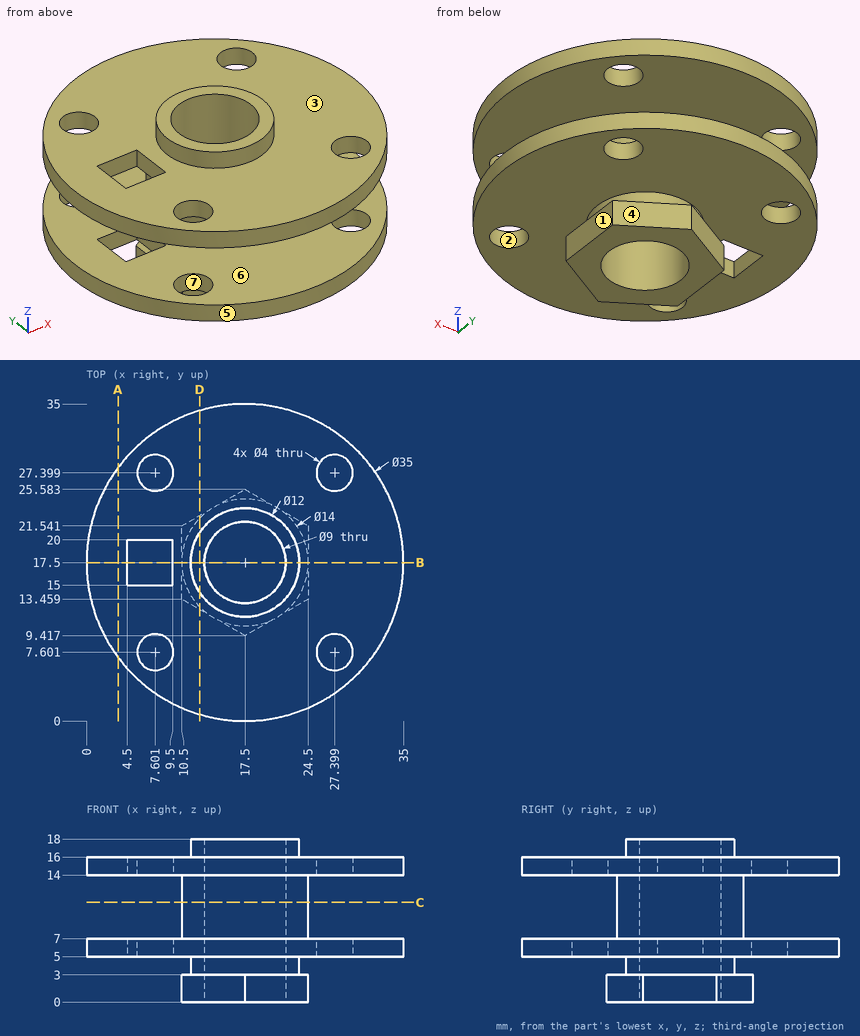
Check sheet for the drawn part. Datum: minimum x, y, z corner. Units: mm. A direction names the side the tool comes from. Coordinates: 2 decimals unless noted, no trailing zeros. Order: outer loops, then holes, each group sorted by start corner. A loop starts at its lowest first (then second) coordinate and runs counter-clockwise, first axis right, second up. Notation, with made-up numbers: M 24.5,56.5 L 28.5,56.5 A21 ccw 28.5,91.5 Z; hole C -36.5,52 d11. An arc over 180 degrees is marked long. One line per question, with ' | ' between items. Start each with the question number.
Item 1: Mould release check, pull along X, two halves, no side actions. Record for the marked faces 5, 6 and 7: pulls with the +X half, pulls with the -X half, needs draft (parallel to the pull), parting line crosses it, or undercut.
Item 2: Sectioned sample at D-D on x = 12.5. Record the cut outline in (y, z).
Item 3: Sectioned sample at C-C on z = 11. Record the cut outline in (x, y).
Item 4: Sectioned sample at B-B on y = 17.5. Count the separate pieces of the cut face and the enclosed holes in it, and give its area (3 significant figures).
Item 5: Material ranges on line 1 (Z direction, x = 29, y = 19.5); line 2 (Y direction, x = 17.5, z = 7.5); line 3 (Y direction, x = 18.5, z = 6.75), recorded low to high.
Item 6: Sectioned sample at A-A on x = 3.5. Record the cut outline in (y, z).
Item 7: Gauge pin test, flat ends, axial feed: P1, Ø12, axis at x = 26, y = 29, coming from the +Z side; P2, Ø0.6, axis at y = 17, z = 6, coming from the -X side; P3, Ø3, axis at x = 5.5, y = 12, coming from the -Z side. Record the tip position at first contact, or that the pin passes through.
Item 8: Access from +Z, -Z, +X, -X, +Y, -Y to the whole of each face (thin tool, end or side, straight path). Record for the marked faces 1, 2, 3 and 4.
Answer below:
1) face 5: parting line crosses it | face 6: needs draft | face 7: undercut
2) outline: M 0.73,5 L 14.18,5 L 14.18,3 L 12.3,3 L 12.3,0 L 22.7,0 L 22.7,3 L 20.82,3 L 20.82,5 L 34.27,5 L 34.27,7 L 22.4,7 L 22.4,14 L 34.27,14 L 34.27,16 L 20.82,16 L 20.82,18 L 14.18,18 L 14.18,16 L 0.73,16 L 0.73,14 L 12.6,14 L 12.6,7 L 0.73,7 Z
3) outline: C 17.5,17.5 d14; hole C 17.5,17.5 d9
4) separate pieces: 4 | enclosed holes: 0 | area: 146 mm^2
5) line 1: z = 5 to 7, 14 to 16 | line 2: y = 10.5 to 13, 22 to 24.5 | line 3: y = 0.03 to 13.11, 21.89 to 34.97
6) outline: M 7,5 L 28,5 L 28,7 L 7,7 Z; M 7,14 L 28,14 L 28,16 L 7,16 Z
7) P1: stops at z = 16 | P2: stops at x = 0 | P3: stops at z = 5
8) face 1: -Z, +X, +Y, -Y | face 2: +Z, -Z | face 3: +Z | face 4: -Z, +X, +Y
